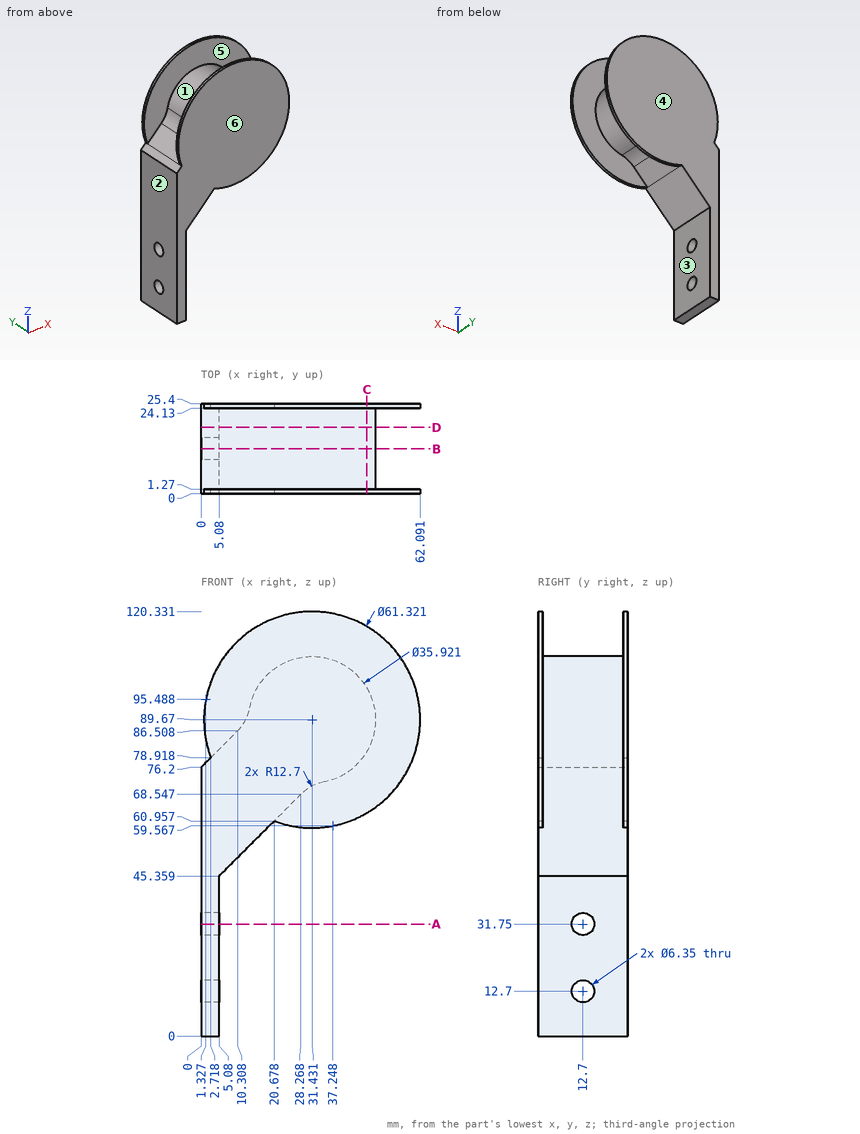
Study the drawing (mm; zero at the part's minimum x, y, z) and answer. A direction names the side the tool comes from. Round coordinates to 2 decimals unless told otherwise and drop trailing zeros. Loops run counter-clockwise (first coordinate to the right, second up) from the corner with the lowest first, then second, coordinate; pieces in that order, holes last. Notation, with made-up numbers: (-3, 49) -> (52, 49) arc R20 ccw to (52, 57) -> close; hole circle Ø2 at (-31, -29). An arc over 180 degrees is marked (long way). One line per item, written item: value.
1) A cutting plane is placed at A-A (z = 31.75). Determine the outline of the cut face in (x, y) (1 decimal).
Answer list:
outline: (0, 0) -> (5.1, 0) -> (5.1, 9.5) -> (0, 9.5) -> close; (0, 15.9) -> (5.1, 15.9) -> (5.1, 25.4) -> (0, 25.4) -> close
2) A cutting plane is placed at B-B (y = 12.7). Determine the outline of the cut face in (x, z) (1 decimal), and give its area (3 significant figures).
Answer list:
outline: (0, 0) -> (5.1, 0) -> (5.1, 9.5) -> (0, 9.5) -> close; (0, 15.9) -> (5.1, 15.9) -> (5.1, 28.6) -> (0, 28.6) -> close; (0, 34.9) -> (5.1, 34.9) -> (5.1, 45.4) -> (28.3, 68.5) arc R12.7 cw to (34.8, 72) arc R18 ccw (long way) to (13.8, 93.1) arc R12.7 cw to (10.3, 86.5) -> (0, 76.2) -> close
area: 1,880 mm²
3) For the marked faces 1, 2 and 3, determine the directions among +Z, -Z, +X, -X, +Y, -Y from which every point of the face is accessible in a straight line to the end or side of a thin tool.
Answer list:
face 1: none
face 2: +Z, -Z, -X, +Y, -Y
face 3: -Z, +X, +Y, -Y
4) A cutting plane is placed at D-D (y = 18.75). Determine the outline of the cut face in (x, z), and give its area (3 significant figures).
Answer list:
outline: (0, 0) -> (5.08, 0) -> (5.08, 45.36) -> (28.27, 68.55) arc R12.7 cw to (34.84, 72.04) arc R17.96 ccw (long way) to (13.8, 93.08) arc R12.7 cw to (10.31, 86.51) -> (0, 76.2) -> close
area: 1,950 mm²
5) Flat-ended cylindrical pins translate along their axes: P1, Ø3, axis at y = 3.5, z = 100, coming from the -X side; P2, Ø4, axis at x = 50, y = 12.5, coming from the -Z side; P3, Ø6, axis at y = 13, z = 92.5, coming from the -X side; P4, Ø5, axis at y = 12.7, z = 12.7, coming from the +X side. Find the tip coordinate at first contact, or state that the pin passes through.
Answer list:
P1: stops at x = 15.79
P2: stops at z = 82.74
P3: stops at x = 12.53
P4: passes through
6) The mould has two halves that part along Y. Classify the marked faces 4, 5 and 6: pulls with the +Y half, pulls with the -Y half, needs draft (parallel to the pull), parting line crosses it, or undercut.
Answer list:
face 4: pulls with the +Y half
face 5: undercut
face 6: pulls with the -Y half
7) A cutting plane is placed at C-C (x = 47). Determine the outline of the cut face in (y, z) (1 decimal).
Answer list:
outline: (0, 63.3) -> (1.3, 63.3) -> (1.3, 80.7) -> (24.1, 80.7) -> (24.1, 63.3) -> (25.4, 63.3) -> (25.4, 116.1) -> (24.1, 116.1) -> (24.1, 98.6) -> (1.3, 98.6) -> (1.3, 116.1) -> (0, 116.1) -> close
8) Consider L1, parallel to Z at x = 1.2, y = 12.7 (1 decimal); L2, parallel to X at y = 21.25, z = 25.5; L3, parallel to Y at x = 36, z = 69.5. Determine where each line is inside the solid, lowest interval first. Write a range as [from, to].
Answer list:
L1: z = [0, 9.5], [15.9, 28.6], [34.9, 77.4]
L2: x = [0, 5.08]
L3: y = [0, 1.27], [24.13, 25.4]
